Can you work these out from the drawing? Everything is in mm from the part's minimum corner. Round coordinates to 2 decimals unless told otherwise and drop trailing zeros. Loops run counter-clockwise (first coordinate to the right, second up) from the corner with the lowest first, then second, coordinate; pieces in that order, holes last. Notation, with made-up numbers: (59.5, 24) - (76.5, 24) arc R13 ccw to (76.5, 40) - close; hole circle Ø1 at (32, -34). An arc over 180 degrees is marked (long way). Put each result on its own line as item: value. Start each with the question number.
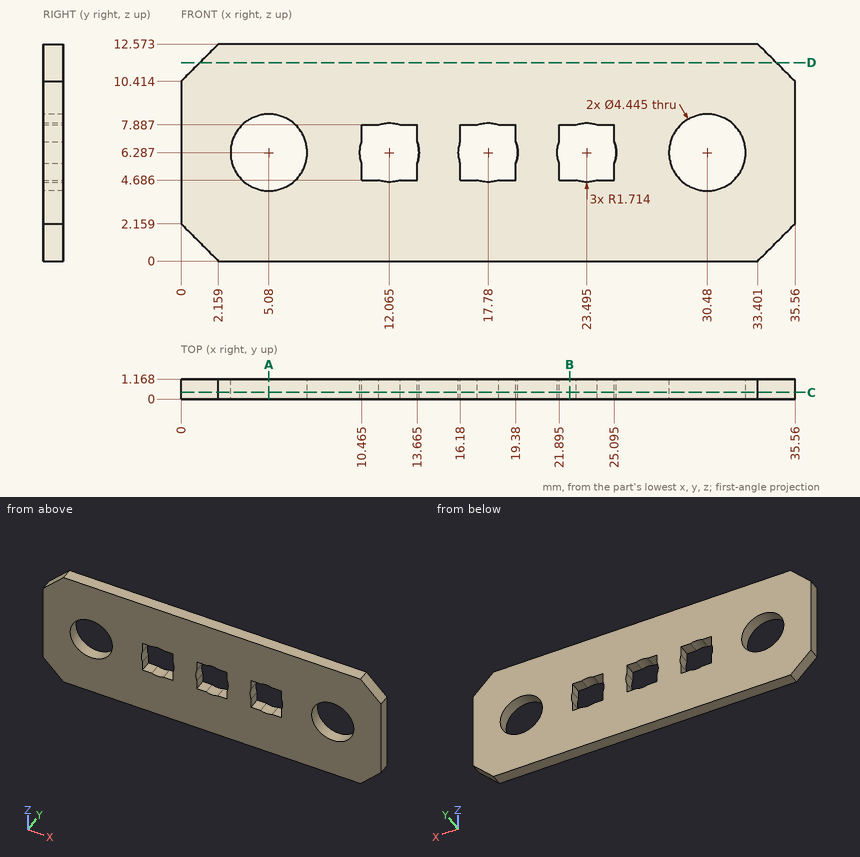
Item 1: Suppose I cut it at A-A, the plane x = 5.08. List the corners of the cut face in (y, z) for me (1 decimal).
Item 2: Suppose I cut it at B-B, the plane x = 22.5. List the corners of the cut face in (y, z) for me.
Item 3: Suppose I cut it at D-D, the plane z = 11.5. List the corners of the cut face in (x, y) for me (1 decimal).
Item 4: Suppose I cut it at C-C, the plane y = 0.4. Count the separate pieces of the cut face and the enclosed holes in it, then the cut area to 3 significant figures.
Item 5: I need wall thicknesses on line 1 (Z direction, x = 30.48, y = 0.3) (1 decimal); line 2 (X direction, y = 0.45, z = 5) (1 decimal); line 3 (Z direction, x = 12, y = 0.55). Which ranges of each line are inside material? Lowest first, please. Write a range as from..to.
Numbers:
1. outline: (0, 0) - (1.2, 0) - (1.2, 4.1) - (0, 4.1) - close; (0, 8.5) - (1.2, 8.5) - (1.2, 12.6) - (0, 12.6) - close
2. outline: (0, 0) - (1.17, 0) - (1.17, 4.69) - (0, 4.69) - close; (0, 7.89) - (1.17, 7.89) - (1.17, 12.57) - (0, 12.57) - close
3. outline: (1.1, 0) - (34.5, 0) - (34.5, 1.2) - (1.1, 1.2) - close
4. separate pieces: 1
4. enclosed holes: 5
4. area: 375 mm^2
5. line 1: 0..4.1, 8.5..12.6
5. line 2: 0..3.3, 6.9..10.5, 13.7..16.2, 19.4..21.9, 25.1..28.7, 32.3..35.6
5. line 3: 0..4.57, 8..12.57
